```python
from build123d import *

# Parameters (mm, degrees)
F0_R          = 206.500881119
F0_R_2        = 19.05
F1_DEPTH      = 3.175
F2_R          = 207.294631119
F2_R_2        = 206.500881119
F3_DEPTH      = 101.6
F3_DEPTH_BACK = 152.4


with BuildPart() as f1:
    # F0 (on Top) → F1 (new body)
    with BuildSketch(Plane.XY):
        Circle(F0_R)
        with BuildLine():
            Line((-203.2, -1.5875), (-22.1682310695, -1.5875))
            ThreePointArc((-22.1682310695, -1.5875), (-15.7154482119, -15.7154482119), (-1.5875, -22.1682310695))
            Line((-1.5875, -22.1682310695), (-1.5875, -203.2))
            ThreePointArc((-1.5875, -203.2), (-143.6884827609, -143.6884827609), (-203.2, -1.5875))
        make_face(mode=Mode.SUBTRACT)
        with BuildLine():
            Line((22.1682310695, -1.5875), (203.2, -1.5875))
            ThreePointArc((203.2, -1.5875), (143.6884827609, -143.6884827609), (1.5875, -203.2))
            Line((1.5875, -203.2), (1.5875, -22.1682310695))
            ThreePointArc((1.5875, -22.1682310695), (15.7154482119, -15.7154482119), (22.1682310695, -1.5875))
        make_face(mode=Mode.SUBTRACT)
        with BuildLine():
            ThreePointArc((-203.2, 1.5875), (-143.6884827609, 143.6884827609), (-1.5875, 203.2))
            Line((-1.5875, 203.2), (-1.5875, 22.1682310695))
            ThreePointArc((-1.5875, 22.1682310695), (-15.7154482119, 15.7154482119), (-22.1682310695, 1.5875))
            Line((-22.1682310695, 1.5875), (-203.2, 1.5875))
        make_face(mode=Mode.SUBTRACT)
        Circle(F0_R_2, mode=Mode.SUBTRACT)
        with BuildLine():
            Line((203.2, 1.5875), (22.1682310695, 1.5875))
            ThreePointArc((22.1682310695, 1.5875), (15.7154482119, 15.7154482119), (1.5875, 22.1682310695))
            Line((1.5875, 22.1682310695), (1.5875, 203.2))
            ThreePointArc((1.5875, 203.2), (143.6884827609, 143.6884827609), (203.2, 1.5875))
        make_face(mode=Mode.SUBTRACT)
    extrude(amount=F1_DEPTH)

    # F2 (on face) → F3 (join, two sides)
    with BuildSketch(Plane.XY.offset(3.175)) as f3_sk:
        Circle(F2_R)
        Circle(F2_R_2, mode=Mode.SUBTRACT)
    extrude(amount=F3_DEPTH)
    extrude(f3_sk.sketch, amount=-F3_DEPTH_BACK)


solid = f1.part
```
Geometry: final body of the model. Coordinates: model frame, mm. A direction names the side the tool comes from. Round coordinates to 2 decimals unless told otherwise and drop trailing zeros. Loops run counter-clockwise (first coordinate to the right, second up) from the corner with the lowest first, then second, coordinate; pieces in that order, holes last. Notation, with made-up numbers: (-5, 48) -> (35, 48) arc R14 cw to (35, 66) -> close; hole circle Ø11 at (9.5, -18). An arc over 180 degrees is marked (long way). Use one line per item in the form item = value. Start each with the question number.
1) Section A-A on x = 51.5. Output: boundary loops of the cut face in (y, z) (1 decimal).
2) Access query for faces 1 (the flat face through (14, -14, 3.175)), 2 (the flat face through (14, -14, 0)), 3 (the cylindrical face through (145.24, -142.12, 1.57)). Directions: +Z, -Z, +X, -X, +Y, -Y. A direction counts if a zero-diameter tool reaches every point of the face in a straight line with its end or side. Return the directions, or none.
3) First-contact query: P1, Ø1.6, axis at x = 89.5, z = 1, coming from the -Y side; P2, Ø1.6, axis at x = -74, z = 1.5, coming from the +Y side; P3, Ø1, axis at x = -70, z = 1, coming from the -Y side. Flat tips, straight axial feed; report the tip coordinate or a pass-through.
4) Draft query along X for faces 4 (the cylindrical face through (15.87, 15.56, 1.57)), 5 (the cylindrical face through (-164.5, -126.14, -20.45)). Return one class per face: released by +X, released by -X, zero draft, split by the parting line, or undercut.
5) Line query: L1, parallel to Y at x = 0, z = -112.5; L2, parallel to Y at x = -80, z = -83; L3, parallel to X at y = 143.5, z = 81.5. Output: solid intervals per line, ascending.
6) Section B-B on y = -137. Output: boundary loops of the cut face in (x, z) (1 decimal).
7) Section C-C on z = -19.5. Output: boundary loops of the cut face in (x, y).
Response:
q1.outline = (-200.8, -149.2) -> (-200, -149.2) -> (-200, 0) -> (-196.6, 0) -> (-196.6, 3.2) -> (-200, 3.2) -> (-200, 104.8) -> (-200.8, 104.8) -> close; (-1.6, 0) -> (1.6, 0) -> (1.6, 3.2) -> (-1.6, 3.2) -> close; (196.6, 0) -> (200, 0) -> (200, -149.2) -> (200.8, -149.2) -> (200.8, 104.8) -> (200, 104.8) -> (200, 3.2) -> (196.6, 3.2) -> close
q2.face_1 = +Z
q2.face_2 = -Z
q2.face_3 = +Z, -Z
q3.P1 = -187.36
q3.P2 = 193.94
q3.P3 = -195.3
q4.face_4 = undercut
q4.face_5 = split by the parting line
q5.L1 = -207.29 to -206.5, 206.5 to 207.29
q5.L2 = -191.24 to -190.37, 190.37 to 191.24
q5.L3 = -149.6 to -148.49, 148.49 to 149.6
q6.outline = (-155.6, -149.2) -> (-154.5, -149.2) -> (-154.5, 0) -> (-150.1, 0) -> (-150.1, 3.2) -> (-154.5, 3.2) -> (-154.5, 104.8) -> (-155.6, 104.8) -> close; (-1.6, 0) -> (1.6, 0) -> (1.6, 3.2) -> (-1.6, 3.2) -> close; (150.1, 0) -> (154.5, 0) -> (154.5, -149.2) -> (155.6, -149.2) -> (155.6, 104.8) -> (154.5, 104.8) -> (154.5, 3.2) -> (150.1, 3.2) -> close
q7.outline = circle Ø414.59 at (0, 0); hole circle Ø413 at (0, 0)
